Work out the finished part from the listing and answer in its coordinate system (mm). Round coordinates to 2 decimals unless told otherwise and drop trailing zeros. Write each loop counter-clockwise with the first axis right and the second up, starting at its lowest first coordinate (ties: lowest second). Pieces come first, ordered by that corner, then holes. Notation, with made-up numbers: (-30, 63.25) -> (11, 63.25) arc R16 ccw to (11, 68.25) -> close; hole circle Ø6 at (46, 29.25). An arc over 180 degrees is marked (long way). Answer as a JSON object with one key per item and string values. Group by question number.
from build123d import *

# Parameters (mm, degrees)
SCHIZZO1_R                   = 30
SCHIZZO1_R_2                 = 21
ESTRUSIONE_ESTRUSIONE1_DEPTH = 4
SCHIZZO2_R                   = 3.05
SCHIZZO3_R                   = 1.5
TAGLIO_ESTRUSIONE1_DEPTH     = 10
RIPETIZIONECIRCOLARE1_COUNT  = 6


with BuildPart() as part:
    # Schizzo1 → Estrusione-Estrusione1 (new body)
    with BuildSketch(Plane.XY):
        Circle(SCHIZZO1_R)
        Circle(SCHIZZO1_R_2, mode=Mode.SUBTRACT)
    extrude(amount=ESTRUSIONE_ESTRUSIONE1_DEPTH)

    # Schizzo2 → Taglia-Rivoluzione1 (revolve, cut)
    with BuildSketch(Plane(origin=(0, 0, 0), x_dir=(0, 0, -1), z_dir=(1, 0, 0))):
        with Locations((-5, 20)):
            Circle(SCHIZZO2_R)
    revolve(axis=Axis((0, 0, 4), (0, 0, -1)), mode=Mode.SUBTRACT)

    # Schizzo3 → Taglio-Estrusione1 (cut)
    with BuildSketch(Plane.XY):
        with Locations((-27.5, 0)):
            Circle(SCHIZZO3_R)
    taglio_estrusione1 = extrude(amount=TAGLIO_ESTRUSIONE1_DEPTH, mode=Mode.SUBTRACT)

    # RipetizioneCircolare1: Taglio-Estrusione1 ×6 about axis
    ripetizionecircolare1_axis = Axis((0, 0, 0), (0, 0, 1))
    for i in range(1, RIPETIZIONECIRCOLARE1_COUNT):
        add(taglio_estrusione1.rotate(ripetizionecircolare1_axis, i * 360 / RIPETIZIONECIRCOLARE1_COUNT), mode=Mode.SUBTRACT)


solid = part.part
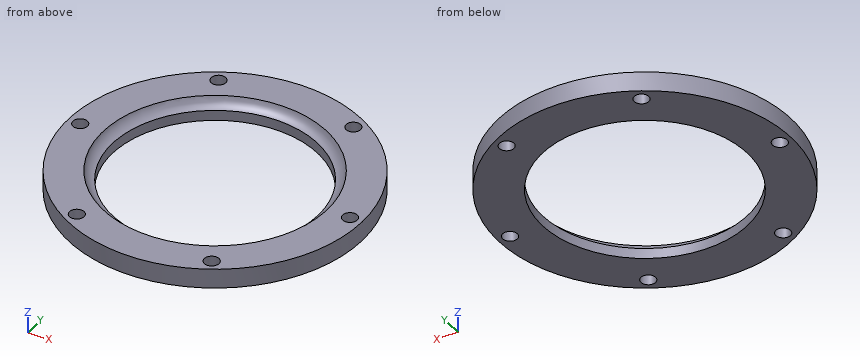
1) Each of these flat-tipped pins is pushed along its axis until it touches: P1, Ø5, axis at x = 27.5, y = 0, coming from the +Z side; P2, Ø1.5, axis at y = 5, z = 1, coming from the -X side. Where does it stop, or does it pass through?
2) A cutting plane is placed at D-D on y = 26.5. Determine the outline of the cut face in (x, z).
3) A cutting plane is placed at A-A on x = 0. Determine the outline of the cut face in (y, z), plus the area to 3 significant figures.
4) A cutting plane is placed at B-B on z = 3. Determine the outline of the cut face in (x, y), plus the area to 3 significant figures.
5) Straight lines are drawn through the part: L1, parallel to Y at x = -13.75, z = 2.4; L2, parallel to Y at x = -13.75, z = 2.95; L3, parallel to X at y = 23, z = 2.05. For each, find the intervals that lie inside material, in ascending order.
6) A cutting plane is placed at C-C on x = -27.5. Determine the outline of the cut face in (y, z), plus the area to 3 significant figures.
Established:
{
 "1": {"P1": "stops at z = 4", "P2": "stops at x = -29.7"},
 "2": {"outline": "(-14.06, 0) -> (14.06, 0) -> (14.06, 4) -> (-14.06, 4) -> close"},
 "3": {"outline": "(-30, 0) -> (-21, 0) -> (-21, 2.12) arc R3.05 cw to (-22.88, 4) -> (-30, 4) -> close; (21, 0) -> (30, 0) -> (30, 4) -> (22.88, 4) arc R3.05 cw to (21, 2.12) -> close", "area": "67.4 mm²"},
 "4": {"outline": "circle Ø60 at (0, 0); hole circle Ø3 at (-27.5, 0); hole circle Ø44.61 at (0, 0); hole circle Ø3 at (-13.75, -23.82); hole circle Ø3 at (-13.75, 23.82); hole circle Ø3 at (13.75, -23.82); hole circle Ø3 at (13.75, 23.82); hole circle Ø3 at (27.5, 0)", "area": "1,220 mm²"},
 "5": {"L1": "y = -26.66 to -25.32, -22.32 to -16.65, 16.65 to 22.32, 25.32 to 26.66", "L2": "y = -26.66 to -25.32, -22.32 to -17.5, 17.5 to 22.32, 25.32 to 26.66", "L3": "x = -19.26 to -15.01, -12.49 to 12.49, 15.01 to 19.26"},
 "6": {"outline": "(-11.99, 0) -> (-1.5, 0) -> (-1.5, 4) -> (-11.99, 4) -> close; (1.5, 0) -> (11.99, 0) -> (11.99, 4) -> (1.5, 4) -> close", "area": "83.9 mm²"}
}
